For this review, take the finished solid that the model builds, in its own axes (mm). Face numbers are marked on the shaded views. A direction names the side the tool comes from. Coordinates: 2 decimals unless noted, no trailing zeros. Order: outer loops, then holes, each group sorted by start corner. A loop starts at its lowest first (then second) coordinate and runs counter-clockwise, first axis right, second up.
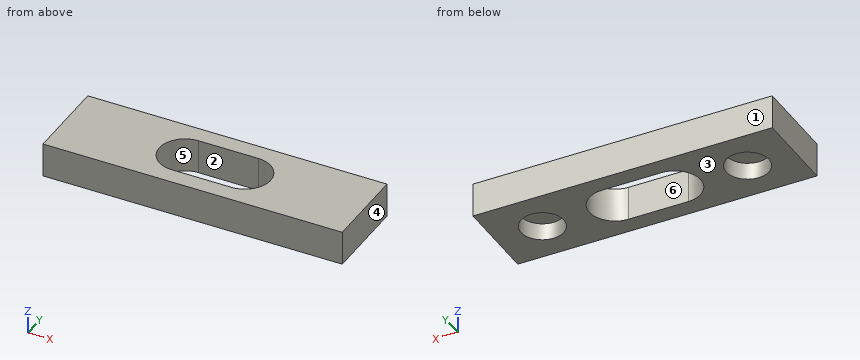
from build123d import *

# Parameters (mm, degrees)
CROQUIS1_W              = 35
CROQUIS1_H              = 10
CROQUIS1_R              = 2.5
SALIENTE_EXTRUIR1_DEPTH = 2
CROQUIS2_W              = 35
CROQUIS2_H              = 10
SALIENTE_EXTRUIR2_DEPTH = 2


with BuildPart() as part:
    # Croquis1 → Saliente-Extruir1 (new body)
    with BuildSketch(Plane.XY):
        with Locations((17.5, 5)):
            Rectangle(CROQUIS1_W, CROQUIS1_H)
        with Locations((29.5, 5)):
            Circle(CROQUIS1_R, mode=Mode.SUBTRACT)
        with Locations((5.5, 5)):
            Circle(CROQUIS1_R, mode=Mode.SUBTRACT)
        with BuildLine():
            Line((14, 8), (21, 8))
            ThreePointArc((21, 8), (24, 5), (21, 2))
            Line((21, 2), (14, 2))
            ThreePointArc((14, 2), (11, 5), (14, 8))
        make_face(mode=Mode.SUBTRACT)
    extrude(amount=SALIENTE_EXTRUIR1_DEPTH)

    # Croquis2 → Saliente-Extruir2 (add)
    with BuildSketch(Plane.XY.offset(2)):
        with Locations((17.5, 5)):
            Rectangle(CROQUIS2_W, CROQUIS2_H)
        with BuildLine():
            Line((14, 8), (21, 8))
            ThreePointArc((21, 8), (24, 5), (21, 2))
            Line((21, 2), (14, 2))
            ThreePointArc((14, 2), (11, 5), (14, 8))
        make_face(mode=Mode.SUBTRACT)
    extrude(amount=SALIENTE_EXTRUIR2_DEPTH)


solid = part.part
1. Take a section at C-C, the plane z = 0.9. Give the boundary of the cut face in (x, y).
Answer below:
outline: (0, 0) - (35, 0) - (35, 10) - (0, 10) - close; hole circle Ø5 at (5.5, 5); hole (14, 2) - (21, 2) arc R3 ccw to (21, 8) - (14, 8) arc R3 ccw to start; hole circle Ø5 at (29.5, 5)
2. To check wall thickness, follow L1, parallel to Y at x = 29.5, z = 1; L2, parallel to Y at x = 20.5, z = 0.95; L3, parallel to X at y = 3.25, z = 2.8. State the ranges of each line that lie inside material, in increasing order.
Answer below:
L1: y = 0 to 2.5, 7.5 to 10
L2: y = 0 to 2, 8 to 10
L3: x = 0 to 11.56, 23.44 to 35
3. Take a section at B-B, the plane z = 2.7. Give the boundary of the cut face in (x, y).
Answer below:
outline: (0, 0) - (35, 0) - (35, 10) - (0, 10) - close; hole (14, 2) - (21, 2) arc R3 ccw to (21, 8) - (14, 8) arc R3 ccw to start
4. Clearance check with a flat-ended pin moving along its axis: pin 1 Ø3 at (x, y) = (6.5, 3) entering from -Z. State where the tip first meets the part, or that it passes through.
Answer below:
pin 1: stops at z = 0
5. Take a section at D-D, the plane x = 13. Give the boundary of the cut face in (y, z).
Answer below:
outline: (0, 0) - (2.17, 0) - (2.17, 4) - (0, 4) - close; (7.83, 0) - (10, 0) - (10, 4) - (7.83, 4) - close
6. Take a section at A-A, the plane y = 5. Give the boundary of the cut face in (x, z).
Answer below:
outline: (0, 0) - (3, 0) - (3, 2) - (8, 2) - (8, 0) - (11, 0) - (11, 4) - (0, 4) - close; (24, 0) - (27, 0) - (27, 2) - (32, 2) - (32, 0) - (35, 0) - (35, 4) - (24, 4) - close
7. Machinability: for the marked faces 1 and 2, which of the approach directions +Z, -Z, +X, -X, +Y, -Y give a long, thin tool a straight path to every point of the face, cutting with its end or side? Answer none if there is none.
Answer below:
face 1: +Z, -Z, +X, -X, +Y
face 2: +Z, -Z
8. The part is to be moulded in two halves that separate along X. For the marked faces 3, 4, 5 and 6, say which applies: +X half, -X half, draft (parallel to the pull), parting line (faces both ways), or undercut.
Answer below:
face 3: draft
face 4: +X half
face 5: undercut
face 6: undercut
